```python
from build123d import *

# Parameters (mm, degrees)
SKETCH1_W           = 215.9
SKETCH1_H           = 57.15
BOSS_EXTRUDE1_DEPTH = 6.35
SKETCH3_W           = 24.892
SKETCH3_H           = 31.242
BOSS_EXTRUDE2_DEPTH = 6.35
SKETCH4_W           = 13.208
SKETCH4_H           = 13.208
CUT_EXTRUDE2_DEPTH  = 124.578309136
SKETCH5_W           = 279.767575851
SKETCH5_H           = 12.7
CUT_EXTRUDE3_DEPTH  = 124.578309136
SKETCH6_W           = 215.9
SKETCH6_H           = 14.45
CUT_EXTRUDE4_DEPTH  = 124.578309136


with BuildPart() as part:
    # Sketch1 → Boss-Extrude1 (new body)
    with BuildSketch(Plane(origin=(0, 0, 0), x_dir=(1, 0, 0), z_dir=(0, 1, 0))):
        Rectangle(SKETCH1_W, SKETCH1_H)
    extrude(amount=BOSS_EXTRUDE1_DEPTH)

    # Sketch3 → Boss-Extrude2 (add)
    with BuildSketch(Plane(origin=(0, 0, 0), x_dir=(1, 0, 0), z_dir=(0, 1, 0))):
        with Locations((-76.2, -44.196)):
            Rectangle(SKETCH3_W, SKETCH3_H)
        with Locations((-38.1, -44.196)):
            Rectangle(SKETCH3_W, SKETCH3_H)
        with Locations((0, -44.196)):
            Rectangle(SKETCH3_W, SKETCH3_H)
        with Locations((38.1, -44.196)):
            Rectangle(SKETCH3_W, SKETCH3_H)
        with Locations((76.2, -44.196)):
            Rectangle(SKETCH3_W, SKETCH3_H)
    extrude(amount=BOSS_EXTRUDE2_DEPTH)

    # Sketch4 → Cut-Extrude2 (cut, through all)
    with BuildSketch(Plane(origin=(0, 0, 0), x_dir=(1, 0, 0), z_dir=(0, 1, 0))):
        with Locations((-107.95, 9.525)):
            Rectangle(SKETCH4_W, SKETCH4_H)
        with Locations((-107.95, -15.875)):
            Rectangle(SKETCH4_W, SKETCH4_H)
        with Locations((107.95, -15.875)):
            Rectangle(SKETCH4_W, SKETCH4_H)
        with Locations((107.95, 9.525)):
            Rectangle(SKETCH4_W, SKETCH4_H)
    extrude(amount=CUT_EXTRUDE2_DEPTH, mode=Mode.SUBTRACT)

    # Sketch5 → Cut-Extrude3 (cut, through all)
    with BuildSketch(Plane(origin=(0, 6.35, 0), x_dir=(1, 0, 0), z_dir=(0, 1, 0))):
        with Locations((31.933787926, 22.225)):
            Rectangle(SKETCH5_W, SKETCH5_H)
    extrude(amount=-CUT_EXTRUDE3_DEPTH, mode=Mode.SUBTRACT)

    # Sketch6 → Cut-Extrude4 (cut, through all)
    with BuildSketch(Plane(origin=(0, 6.35, 0), x_dir=(1, 0, 0), z_dir=(0, 1, 0))):
        with Locations((0, 8.65)):
            Rectangle(SKETCH6_W, SKETCH6_H)
    extrude(amount=-CUT_EXTRUDE4_DEPTH, mode=Mode.SUBTRACT)


solid = part.part
```
Geometry: final body of the model. Coordinates: model frame, mm. A direction names the side the tool comes from. Coordinates: 2 decimals unless noted, no trailing zeros. Order: outer loops, then holes, each group sorted by start corner. A loop starts at its lowest first (then second) coordinate and runs counter-clockwise, first axis right, second up. Notation, with made-up numbers: (-21, 27) -> (4, 27) arc R14 ccw to (4, 53) -> close; hole circle Ø2 at (27, 60.5). An arc over 180 degrees is marked (long way). Use CSV: the item, a comma, the result in double quotes.
1) Section D-D on z = 19. Output: boundary loops of the cut face in (x, y), then the cut area to 3 significant figures.
Findings:
outline,"(-101.35, 0) -> (101.35, 0) -> (101.35, 6.35) -> (-101.35, 6.35) -> close"
area,"1,290 mm^2"
2) Section A-A on z = 41.5. Output: boundary loops of the cut face in (x, y).
Findings:
outline,"(-88.65, 0) -> (-63.75, 0) -> (-63.75, 6.35) -> (-88.65, 6.35) -> close; (-50.55, 0) -> (-25.65, 0) -> (-25.65, 6.35) -> (-50.55, 6.35) -> close; (-12.45, 0) -> (12.45, 0) -> (12.45, 6.35) -> (-12.45, 6.35) -> close; (25.65, 0) -> (50.55, 0) -> (50.55, 6.35) -> (25.65, 6.35) -> close; (63.75, 0) -> (88.65, 0) -> (88.65, 6.35) -> (63.75, 6.35) -> close"
3) Pin query (flat end, axial travel): pin 1 Ø3 at (y, z) = (2.5, 48.5) entering from -X; pin 2 Ø3 at (x, y) = (-104.5, 4.5) entering from +Z (3 decimals); pin 3 Ø1.9 at (y, z) = (2.5, 37) entering from +X; pin 4 Ø1.5 at (x, z) = (83, 51.5) entering from -Y. Return the tip coordinate at first contact, or that it passes through.
Findings:
pin 1,"stops at x = -88.65"
pin 2,"stops at z = 28.575"
pin 3,"stops at x = 88.65"
pin 4,"stops at y = 0"
4) Line query: line 1 (X direction, y = 6.25, z = 37.5); line 2 (X direction, y = 1.5, z = 19.5); line 3 (Z direction, x = 51, y = 0.5) (3 decimals). Output: solid intervals per line, ascending.
Findings:
line 1,"x = -88.65 to -63.75, -50.55 to -25.65, -12.45 to 12.45, 25.65 to 50.55, 63.75 to 88.65"
line 2,"x = -101.35 to 101.35"
line 3,"z = -1.425 to 28.575"
5) Access query for faces 1 (the flat face through (-25.654, 3, 44)), 2 (the flat face through (88.646, 3, 44)), 3 (the flat face through (105, 3, 22.479)), 4 (the flat face through (-105, 3, 9.271)), 5 (the flat face through (-2, 6.35, 22)). Directions: +Z, -Z, +X, -X, +Y, -Y. A direction counts if a zero-diameter tool reaches every point of the face in a straight line with its end or side. Return the directions, or none.
Findings:
face 1,"+Z, +Y, -Y"
face 2,"+Z, +X, +Y, -Y"
face 3,"+X, +Y, -Y"
face 4,"-X, +Y, -Y"
face 5,"+Z, -Z, +X, -X, +Y"
6) Mould query, pull axis Z, two halves, no side actions, for faces 6 (the flat face through (-107.95, 3, 4)), 7 (the flat face through (101.346, 3, 16)), 8 (the flat face through (-57, 3, 28.575)). Classes: +Z half, -Z half, draft (parallel to the pull), parting line (faces both ways), or undercut.
Findings:
face 6,"draft"
face 7,"undercut"
face 8,"+Z half"
7) Section C-C on x = 23.5. Output: boundary loops of the cut face in (y, z) (3 decimals).
Findings:
outline,"(0, -1.425) -> (6.35, -1.425) -> (6.35, 28.575) -> (0, 28.575) -> close"
